```python
from build123d import *

# Parameters (mm, degrees)
F0_W          = 19.2
F0_H          = 100
F1_DEPTH      = 19.2
F2_W          = 15.4
F2_H          = 15.4
F3_DEPTH      = 18
F5_DEPTH      = 7.7
F5_DEPTH_BACK = 7.7
F6_SIZE       = 0.5


# Not quite as in the source:
# - a pattern or mirror of a feature is missing from the dataset's text; its kind, count and spacing are read off the source's solid


with BuildPart() as f1:
    # F0 (on Top) → F1 (new body)
    with BuildSketch(Plane.XY):
        Rectangle(F0_W, F0_H)
    extrude(amount=F1_DEPTH)

    # F2 (on face) → F3 (cut)
    with BuildSketch(Plane.YZ.offset(9.6)):
        with Locations((-40.4, 9.6)):
            Rectangle(F2_W, F2_H)
    f3 = extrude(amount=-F3_DEPTH, mode=Mode.SUBTRACT)

    # F3_copies: F3 across plane
    add(f3.mirror(Plane.ZX), mode=Mode.SUBTRACT)

    # F4 (on Right) → F5 (cut, two sides)
    with BuildSketch(Plane.YZ) as f5_sk:
        Polygon((1.3316043909, 1.4935935394), (8, 5.3435935394), (14.6683956091, 9.1935935394), (-10.4682390124, 52.7315218353), (-23.8050302307, 45.0315218353), align=None)
    extrude(amount=-F5_DEPTH, mode=Mode.SUBTRACT)
    extrude(f5_sk.sketch, amount=F5_DEPTH_BACK, mode=Mode.SUBTRACT)

    # F6
    f6_edges = [f1.edges().sort_by_distance(p)[0] for p in [
        (-9.6, 50, 9.6),
        (-9.6, -50, 9.6),
        (-9.6, 0, 0),
        (-9.6, 0, 19.2),
        (9.6, -50, 9.6),
        (0, -50, 0),
        (0, -50, 19.2),
        (9.6, 50, 9.6),
        (0, 50, 0),
        (0, 50, 19.2),
        (9.6, 0, 0),
        (9.6, 0, 19.2),
    ]]
    chamfer(f6_edges, length=F6_SIZE)


solid = f1.part
```
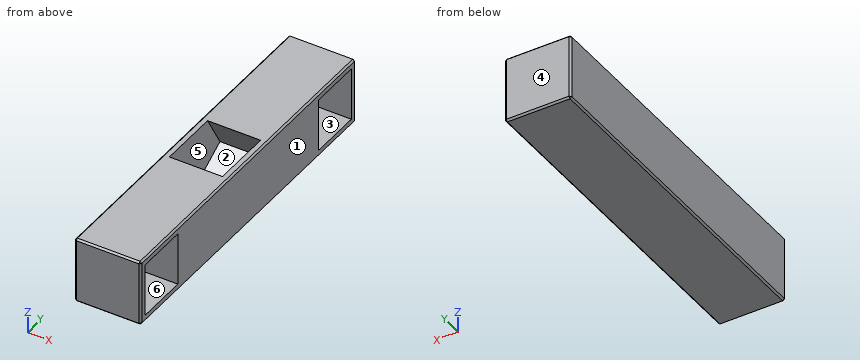
Can you work these out from the model? Positions are in its coordinate system, mm. Face numbers are marked on the shaded views. A direction names the side the tool comes from. Give positions to 0.01 mm unless a question says otherwise; leave off trailing zeros. Order: outer loops, then holes, each group sorted by start corner. A loop starts at its lowest first (then second) coordinate and runs counter-clockwise, first axis right, second up. Notation, with made-up numbers: M 53,70 L 109,70 A19 cw 109,93 Z; hole C 51.25,31 d1. An arc over 180 degrees is marked long. Write item = value, one per line. Start each with the question number.
Q1. Will these pins go through, and if not, where does the flat tip stop? pin 1 Ø1 at (y, z) = (39, 17) entering from +X; pin 2 Ø3 at (x, y) = (-1.5, 2) entering from +Z; pin 3 Ø4.5 at (y, z) = (43, 9.5) entering from +X.
Q2. Suppose I cut it at B-B (y = -44). Write out the boundary of the cut face in (x, z), plus the area to 3 significant figures.
Q3. I need wall thicknesses on probe 1 along Y at (x, z) = (8.5, 15.5); probe 2 along X at (y, z) = (9.5, 15.5); probe 3 along Y at (x, z) = (-5, 3). Which ranges of each line are inside material? Lowest first, please. Write a range as [from, to].
Q4. We'd pull the mould along X, two halves only. Please class the marked faces 1, 2 and 3: pulls with the +X half, pulls with the -X half, needs draft (parallel to the pull), parting line crosses it, or undercut.
Q5. Suppose I cut it at D-D (y = 11.5). Write out the boundary of the cut face in (x, z).
Q6. For the marked faces 4, 5 and 6, which set-ups out of +Z, -Z, +X, -X, +Y, -Y let a thin tool reach every point of the face, with its end or its side?
Q7. Suppose I cut it at C-C (z = 8). Write out the boundary of the cut face in (x, y), plus the area to 3 significant figures.
Q8. Suppose I cut it at A-A (x = -5). Write out the boundary of the cut face in (y, z), plus the area to 3 significant figures.
Check result:
q1.pin_1 = 9.6
q1.pin_2 = 2.93
q1.pin_3 = -8.4
q2.outline = M -9.6,0.5 L -9.1,0 L 9.1,0 L 9.6,0.5 L 9.6,1.9 L -8.4,1.9 L -8.4,17.3 L 9.6,17.3 L 9.6,18.7 L 9.1,19.2 L -9.1,19.2 L -9.6,18.7 Z
q2.area = 90.9 mm2
q3.probe_1 = [-50, -48.1], [-32.7, 32.7], [48.1, 50]
q3.probe_2 = [-9.6, -7.7], [7.7, 9.6]
q3.probe_3 = [-50, -48.1], [-32.7, 0.46], [3.94, 32.7], [48.1, 50]
q4.face_1 = pulls with the +X half
q4.face_2 = undercut
q4.face_3 = needs draft
q5.outline = M -9.6,0.5 L -9.1,0 L 9.1,0 L 9.6,0.5 L 9.6,18.7 L 9.1,19.2 L -9.1,19.2 L -9.6,18.7 Z; hole M -7.7,7.36 L 7.7,7.36 L 7.7,14.68 L -7.7,14.68 Z
q6.face_4 = +Z, -Z, +X, -X, +Y
q6.face_5 = none
q6.face_6 = +X
q7.outline = M -9.6,-49.5 L -9.1,-50 L 9.1,-50 L 9.6,-49.5 L 9.6,-48.1 L -8.4,-48.1 L -8.4,-32.7 L 9.6,-32.7 L 9.6,32.7 L -8.4,32.7 L -8.4,48.1 L 9.6,48.1 L 9.6,49.5 L 9.1,50 L -9.1,50 L -9.6,49.5 Z; hole M -7.7,-2.42 L 7.7,-2.42 L 7.7,12.6 L -7.7,12.6 Z
q7.area = 1,130 mm2
q8.outline = M -50,0.5 L -49.5,0 L 49.5,0 L 50,0.5 L 50,18.7 L 49.5,19.2 L 8.89,19.2 L 14.67,9.19 L 1.33,1.49 L -8.89,19.2 L -49.5,19.2 L -50,18.7 Z; hole M -48.1,1.9 L -32.7,1.9 L -32.7,17.3 L -48.1,17.3 Z; hole M 32.7,1.9 L 48.1,1.9 L 48.1,17.3 L 32.7,17.3 Z
q8.area = 1,200 mm2
